from build123d import *

# Parameters (mm, degrees)
SKETCH1_R           = 1.6
SKETCH1_W           = 1
SKETCH1_H           = 27
BOSS_EXTRUDE1_DEPTH = 3
SKETCH1_3_W         = 1
SKETCH1_3_H         = 27
BOSS_EXTRUDE2_DEPTH = 5
BOSS_EXTRUDE3_DEPTH = 101
SKETCH2_R           = 2.25
CUT_EXTRUDE1_DEPTH  = 1.5
SKETCH4_R           = 2.25
CUT_EXTRUDE2_DEPTH  = 1.5
SKETCH5_R           = 1.6
CUT_EXTRUDE3_DEPTH  = 3
SKETCH6_R           = 2.25
CUT_EXTRUDE4_DEPTH  = 1.5
SKETCH7_W           = 16.5
SKETCH7_H           = 98
CUT_EXTRUDE5_DEPTH  = 3
SKETCH8_W           = 16.5
SKETCH8_H           = 14.6
CUT_EXTRUDE6_DEPTH  = 3
FILLET1_R           = 10
FILLET2_R           = 10
FILLET3_R           = 10
SKETCH9_W           = 67.5
SKETCH9_H           = 22
SKETCH9_W_2         = 8
CUT_EXTRUDE7_DEPTH  = 10
FILLET4_R           = 3
SKETCH10_W          = 70.5
SKETCH10_H          = 88
SKETCH10_W_2        = 6
CUT_EXTRUDE8_DEPTH  = 10
FILLET5_R           = 3


# Some blends are built 0.0001 mm under size
with BuildPart() as part:
    # Sketch1 → Boss-Extrude1 (new body)
    # profile 1 of 3: a face of its own
    with BuildSketch(Plane.XY):
        Polygon((0, 3), (0, 0), (117, 0), (117, 3), (17.5, 3), (16.5, 3), align=None)
    # profile 2 of 3: a face of its own
    with BuildSketch(Plane.XY):
        Polygon((0, 35), (0, 3), (16.5, 3), (16.5, 30), (17.5, 30), (17.5, 3), (117, 3), (117, 35), align=None)
        with Locations((10, 10.2)):
            Circle(SKETCH1_R, mode=Mode.SUBTRACT)
        with Locations((37.5, 13.5)):
            Circle(SKETCH1_R, mode=Mode.SUBTRACT)
        with Locations((37.5, 31.5)):
            Circle(SKETCH1_R, mode=Mode.SUBTRACT)
    # profile 3 of 3: a face of its own
    with BuildSketch(Plane.XY):
        with Locations((17, 16.5)):
            Rectangle(SKETCH1_W, SKETCH1_H)
    extrude(amount=BOSS_EXTRUDE1_DEPTH)

    # Sketch1<3> → Boss-Extrude2 (add)
    with BuildSketch(Plane.XY):
        with Locations((17, 16.5)):
            Rectangle(SKETCH1_3_W, SKETCH1_3_H)
    extrude(amount=BOSS_EXTRUDE2_DEPTH)

    # Sketch1<7> → Boss-Extrude3 (add)
    with BuildSketch(Plane.XY):
        Polygon((0, 3), (0, 0), (117, 0), (117, 3), (17.5, 3), (16.5, 3), align=None)
    extrude(amount=BOSS_EXTRUDE3_DEPTH)

    # Sketch2 → Cut-Extrude1 (cut)
    with BuildSketch(Plane(origin=(0, 0, 0), x_dir=(-1, 0, 0), z_dir=(0, 0, -1))):
        with Locations((-37.5, 31.5)):
            Circle(SKETCH2_R)
        with Locations((-37.5, 13.5)):
            Circle(SKETCH2_R)
    extrude(amount=-CUT_EXTRUDE1_DEPTH, mode=Mode.SUBTRACT)

    # Sketch4 → Cut-Extrude2 (cut)
    with BuildSketch(Plane.XY.offset(3)):
        with Locations((10, 10.2)):
            Circle(SKETCH4_R)
    extrude(amount=-CUT_EXTRUDE2_DEPTH, mode=Mode.SUBTRACT)

    # Sketch5 → Cut-Extrude3 (cut)
    with BuildSketch(Plane(origin=(0, 3, 0), x_dir=(1, 0, 0), z_dir=(0, 1, 0))):
        with Locations(Location((34.5, -12, 0), (0, 0, 270))):
            Circle(SKETCH5_R)
        with Locations(Location((34.5, -92, 0), (0, 0, 270))):
            Circle(SKETCH5_R)
    extrude(amount=-CUT_EXTRUDE3_DEPTH, mode=Mode.SUBTRACT)

    # Sketch6 → Cut-Extrude4 (cut)
    with BuildSketch(Plane.XZ):
        with Locations(Location((34.5, 92, 0), (0, 0, 270))):
            Circle(SKETCH6_R)
        with Locations(Location((34.5, 12, 0), (0, 0, 270))):
            Circle(SKETCH6_R)
    extrude(amount=-CUT_EXTRUDE4_DEPTH, mode=Mode.SUBTRACT)

    # Sketch7 → Cut-Extrude5 (cut)
    with BuildSketch(Plane(origin=(0, 3, 0), x_dir=(1, 0, 0), z_dir=(0, 1, 0))):
        with Locations((8.25, -52)):
            Rectangle(SKETCH7_W, SKETCH7_H)
    extrude(amount=-CUT_EXTRUDE5_DEPTH, mode=Mode.SUBTRACT)

    # Sketch8 → Cut-Extrude6 (cut)
    with BuildSketch(Plane.XY.offset(3)):
        with Locations((8.25, 27.7)):
            Rectangle(SKETCH8_W, SKETCH8_H)
    extrude(amount=-CUT_EXTRUDE6_DEPTH, mode=Mode.SUBTRACT)

    # Fillet1
    fillet1_edges = [part.edges().sort_by_distance(p)[0] for p in [
        (0, 20.4, 1.5),
    ]]
    fillet(fillet1_edges, radius=FILLET1_R)

    # Fillet2
    fillet2_edges = [part.edges().sort_by_distance(p)[0] for p in [
        (0, 0, 1.5),
    ]]
    fillet(fillet2_edges, radius=FILLET2_R)

    # Fillet3
    # the kernel refuses this fillet: 10 mm, written as the material it takes off along each edge
    with BuildSketch(Plane(origin=(1.5, 30, 5), x_dir=(0, 0, -1), z_dir=(1, 0, 0))) as fillet3_piece_1:
        with BuildLine():
            CenterArc((10, -6), FILLET3_R, 143.130102354, 36.869897646)
            Line((0, -6), (-0.2, -6))
            Line((-0.2, -6), (-0.2, 0))
            Line((-0.2, 0), (0, 0.2))
            ThreePointArc((0, 0.2), (1, 0.2), (1.84, 0.12))
            Line((1.84, 0.12), (2, 0))
        make_face()
    extrude(amount=31, mode=Mode.SUBTRACT)

    # Sketch9 → Cut-Extrude7 (cut)
    with BuildSketch(Plane.XY.offset(3)):
        with Locations((78.25, 19)):
            Rectangle(SKETCH9_W, SKETCH9_H)
        with Locations((26.5, 19)):
            Rectangle(SKETCH9_W_2, SKETCH9_H)
    extrude(amount=-CUT_EXTRUDE7_DEPTH, mode=Mode.SUBTRACT)

    # Fillet4
    fillet4_edges = [part.edges().sort_by_distance(p)[0] for p in [
        (44.5, 8, 1.5),
        (44.5, 30, 1.5),
        (112, 30, 1.5),
        (112, 8, 1.5),
        (22.5, 8, 1.5),
        (22.5, 30, 1.5),
        (30.5, 30, 1.5),
        (30.5, 8, 1.5),
    ]]
    fillet(fillet4_edges, radius=FILLET4_R)

    # Sketch10 → Cut-Extrude8 (cut)
    with BuildSketch(Plane(origin=(0, 3, 0), x_dir=(1, 0, 0), z_dir=(0, 1, 0))):
        with Locations((76.75, -52)):
            Rectangle(SKETCH10_W, SKETCH10_H)
        with Locations((24.5, -52)):
            Rectangle(SKETCH10_W_2, SKETCH10_H)
    extrude(amount=-CUT_EXTRUDE8_DEPTH, mode=Mode.SUBTRACT)

    # Fillet5
    fillet5_edges = [part.edges().sort_by_distance(p)[0] for p in [
        (41.5, 1.5, 96),
        (41.5, 1.5, 8),
        (112, 1.5, 8),
        (112, 1.5, 96),
        (21.5, 1.5, 96),
        (21.5, 1.5, 8),
        (27.5, 1.5, 8),
        (27.5, 1.5, 96),
    ]]
    fillet(fillet5_edges, radius=FILLET5_R - 0.0001)  # a hair under: the kernel refuses the full size


solid = part.part
Work out the finished part from the listing and answer in its coordinate system (mm). A direction names the side the tool comes from. Give positions to 0.01 mm unless a question says otherwise; leave off trailing zeros. Write each loop counter-clockwise with the first axis right and the second up, starting at its lowest first coordinate (ties: lowest second). Pieces come first, ordered by that corner, then holes.
Q1. For a pull along Y with two mould halves and no side action, classify faces 1 (the face through (44.5, 19, 2)), 2 (the face through (34, 1.5, 94)), 3 (the face through (111.14, 1.48, 8.9)), 4 (the face through (10, 12, 1.5)) as released by +Y, released by -Y, zero draft, split by the parting line, or undercut.
Answer:
face 1: undercut
face 2: released by -Y
face 3: zero draft
face 4: undercut
Q2. The part is cut by section B-B on z = 42. Give the vertices of the cut face in (x, y).
Answer:
outline: (16.5, 0) - (21.5, 0) - (21.5, 3) - (16.5, 3) - close; (27.5, 0) - (41.5, 0) - (41.5, 3) - (27.5, 3) - close; (112, 0) - (117, 0) - (117, 3) - (112, 3) - close
Q3. A tool of negligible diameter and unlimited length cuts with its end or side. For faces 5 (the face through (45.4, 29.14, 1.48)), 6 (the face through (76, 2, 96)), 7 (the face through (8, 13, 3)), 8 (the face through (36.5, 30, 1.5)), from which of +Z, -Z, +X, -X, +Y, -Y can it reach the whole face along a straight path? Write none if from no direction.
Answer:
face 5: +Z, -Z
face 6: +Y, -Y
face 7: +Z, -X, +Y, -Y
face 8: -Z
Q4. The part is cut by section C-C on x = 54.5. Give the vertices of the cut face in (y, z), and give its area (3 significant figures).
Answer:
outline: (0, 0) - (8, 0) - (8, 3) - (3, 3) - (3, 8) - (0, 8) - close; (0, 96) - (3, 96) - (3, 101) - (0, 101) - close; (30, 0) - (35, 0) - (35, 3) - (30, 3) - close
area: 69.0 mm2
Q5. Straight lines are drawn through the part: L1, parallel to Y at x = 37.5, z = 0.7; L2, parallel to Y at x = 37.5, z = 2.4; L3, parallel to X at y = 1, z = 92. For each, find the intervals that lie inside material, in ascending order.
Answer:
L1: y = 0 to 11.25, 15.75 to 29.25, 33.75 to 35
L2: y = 0 to 11.9, 15.1 to 29.9, 33.1 to 35
L3: x = 16.5 to 21.5, 27.5 to 32.25, 36.75 to 41.5, 112 to 117
Q6. Given pin 1 (1.3 mm diameter, centred on x = 37.5, y = 14, fed in from -Z); pin 2 (1.5 mm diameter, centred on y = 1, z = 52.5, fed in from -X); pin 3 (13 mm diameter, centred on x = 9.5, y = 8.5, fed in from +Z); pin 4 (6 mm diameter, centred on x = 45.5, y = 20.5, fed in from -Z), each flat-ended and moving along its own axis, determine where each tip first touches the part or whether it passes through.
Answer:
pin 1: passes through
pin 2: stops at x = 16.5
pin 3: stops at z = 3
pin 4: stops at z = 0
Q7. The part is cut by section A-A on y = 31.5. Give the vertices of the cut face in (x, z).
Answer:
outline: (16.5, 0) - (35.25, 0) - (35.25, 1.5) - (35.9, 1.5) - (35.9, 3) - (16.5, 3) - close; (39.1, 1.5) - (39.75, 1.5) - (39.75, 0) - (117, 0) - (117, 3) - (39.1, 3) - close
